The figure shows three views and two pictorial views of one solid part (mm, origin at its lowest corner). Answer the questions. A direction names the side the tool comes from. Give positions to 0.01 mm unless a question says otherwise; leave off trailing zeros. Loops run counter-clockwise (first coordinate to the right, second up) from the corner with the lowest first, then second, coordinate; pieces in that order, holes last. Notation, with made-up numbers: (24, 23) - (46, 23) arc R30 ccw to (46, 54) - close; hole circle Ø5 at (76.25, -11.5). An arc over 180 degrees is marked (long way). Use a Markdown table: item, result. Add a question column.
Item 1: Which of the six approach directions +Z, -Z, +X, -X, +Y, -Y give full straight-line access (tool end or side, diameter ignored) to the marked faces 1, 2, 3 and 4?
Item 2: For a pull along Y with two mould halves and no side action, classify the marked faces 5, 6, 7 and 8 as +Y half, -Y half, draft (parallel to the pull), parting line (faces both ways), or undercut.
Item 3: Consider probe 1 along Y at (x, z) = (15.75, 12.5); probe 2 along Z at (x, y) = (23.25, 22.25). Determine where each line is inside the solid, lowest interval first. Write a range as [from, to].
Item 4: A cutting plane is placed at B-B (x = 17.5). Determine the outline of the cut face in (y, z), plus the area to 3 significant figures.
Item 5: A cutting plane is placed at D-D (y = 27.5). Determine the outline of the cut face in (x, z), plus the area to 3 significant figures.
Item 6: Each of these flat-tipped pins is pushed along its axis until it touches: P1, Ø10, axis at y = 16, z = 13.5, coming from the -X side; P2, Ø1, axis at x = 20, z = 10.5, coming from the -Y side; P3, Ø10, axis at x = 19, z = 8.5, coming from the +Y side. Where does it stop, or does it pass through?
Item 7: A cutting plane is placed at A-A (z = 17.5). Determine the outline of the cut face in (x, y), plus the area to 3 significant figures.
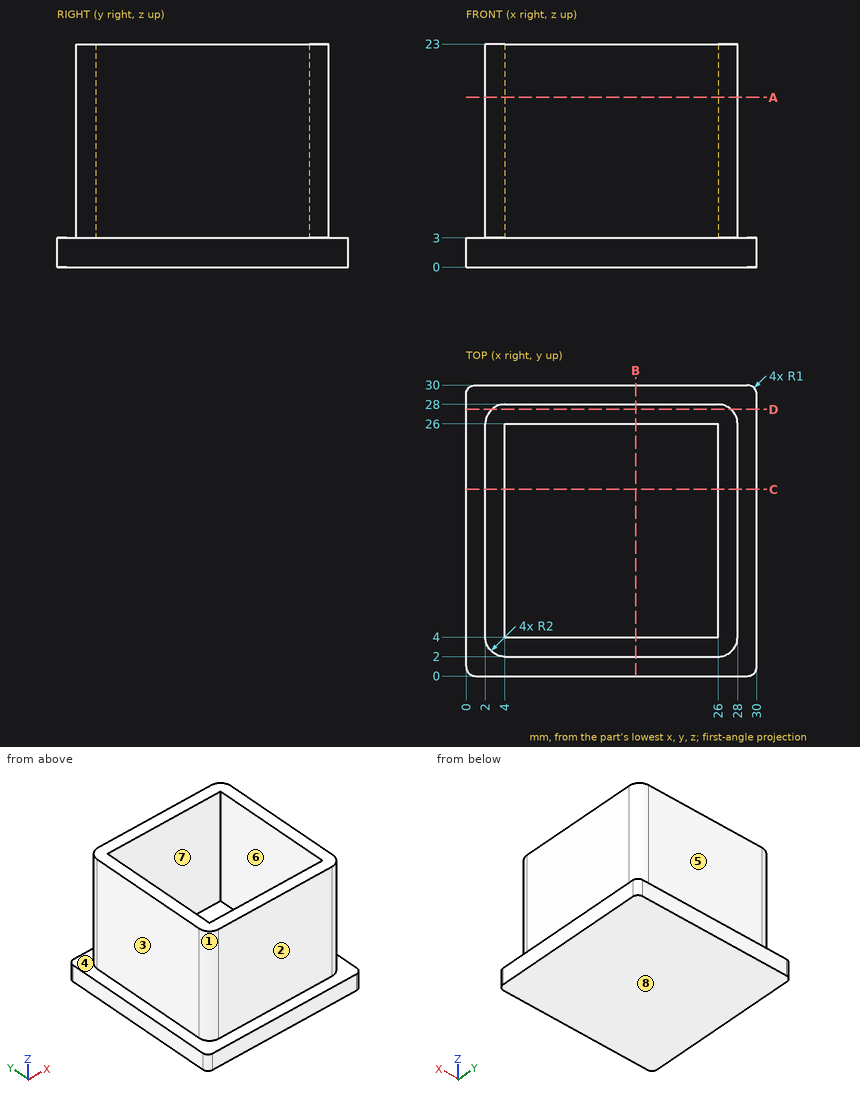
Geometry says:
| question | item | result |
|---|---|---|
| 1 | face 1 | +Z, -X, -Y |
| 1 | face 2 | +Z, +X, -X, -Y |
| 1 | face 3 | +Z, -X, +Y, -Y |
| 1 | face 4 | +Z |
| 2 | face 5 | +Y half |
| 2 | face 6 | undercut |
| 2 | face 7 | undercut |
| 2 | face 8 | draft |
| 3 | probe 1 | [2, 4], [26, 28] |
| 3 | probe 2 | [0, 3] |
| 4 | outline | (0, 0) - (30, 0) - (30, 3) - (28, 3) - (28, 23) - (26, 23) - (26, 3) - (4, 3) - (4, 23) - (2, 23) - (2, 3) - (0, 3) - close |
| 4 | area | 170 mm² |
| 5 | outline | (0, 0) - (30, 0) - (30, 3) - (27.32, 3) - (27.32, 23) - (2.68, 23) - (2.68, 3) - (0, 3) - close |
| 5 | area | 583 mm² |
| 6 | P1 | x = 2 |
| 6 | P2 | y = 2 |
| 6 | P3 | y = 28 |
| 7 | outline | (2, 4) arc R2 ccw to (4, 2) - (26, 2) arc R2 ccw to (28, 4) - (28, 26) arc R2 ccw to (26, 28) - (4, 28) arc R2 ccw to (2, 26) - close; hole (4, 4) - (26, 4) - (26, 26) - (4, 26) - close |
| 7 | area | 189 mm² |
